```python
from build123d import *

# Parameters (mm, degrees)
BOSS_EXTRUDE1_DEPTH  = 19.9517
M3_CLEARANCE_HOLE1_D = 3.4


with BuildPart() as part:
    # Sketch1 → Boss-Extrude1 (new body)
    with BuildSketch(Plane(origin=(0, 0, 0), x_dir=(1, 0, 0), z_dir=(0, 1, 0))):
        Polygon((16.637, 24.92375), (26.67, 24.92375), (26.67, -24.92375), (16.637, -24.92375), (16.637, -32.03575), (-1.143, -32.03575), (-1.143, -24.92375), (-26.67, -24.92375), (-26.67, 24.92375), (-1.143, 24.92375), (-1.143, 32.03575), (16.637, 32.03575), align=None)
    extrude(amount=BOSS_EXTRUDE1_DEPTH)

    # M3 Clearance Hole1 (through all)
    with Locations(Plane(origin=(0, 19.9517, 0), x_dir=(1, 0, 0), z_dir=(0, 1, 0))):
        with Locations((7.747, 28.86075), (7.747, -28.86075)):
            Hole(M3_CLEARANCE_HOLE1_D / 2)


solid = part.part
```
Could you check a few things on this model? Use its own coordinates, in mm. A direction names the side the tool comes from. Round coordinates to 2 decimals unless told otherwise and drop trailing zeros. Write each loop counter-clockwise with the first axis right and the second up, starting at its lowest first coordinate (ties: lowest second). Pieces come first, ordered by that corner, then holes. Notation, with made-up numbers: M 46.25,37.25 L 81.25,37.25 A23 ccw 81.25,53.25 Z; hole C 24.25,60 d10. An arc over 180 degrees is marked long. Write each question's results on one line, items separated by ' | '. Start each with the question number.
1. Imagine slicing it at D-D on z = -26. List the corners of the cut face in (x, y) for me.
2. Imagine slicing it at C-C on x = -9. List the corners of the cut face in (y, z) for me, and give its area (3 significant figures).
3. I'm going to push flat-ended pins straight in: pin 1 Ø10 at (x, y) = (-19, 9.5) entering from -Z; pin 2 Ø10 at (x, y) = (-11, 14.5) entering from +Z; pin 3 Ø8 at (y, z) = (8.5, -29.5) entering from -X. Where does each tip first touch, or does it pass through?
4. I need wall thicknesses on L1, parallel to Z at x = 8, y = 16; L2, parallel to X at y = 1.5, z = 26.5; L3, parallel to Z at x = -23.5, y = 5.75. Which ranges of each line are inside material? Lowest first, please. Write a range as from..to.
5. Thinking about a two-plate mould opening in X: for faces 6 (the face through (6.83, 9.84, 27.43)), 7 (the face through (-1.143, 10, -28)), 8 (the face through (-14, 10, -24.924)), 9 (the face through (16.637, 10, 28)), which applies, +X half, -X half, draft (parallel to the pull), parting line (faces both ways), or undercut?
6. On a 3-axis mill with a long thin cutter (end or side, diameter ignored), from which of +Z, -Z, +X, -X, +Y, -Y can I reach the whole of each face in a straight line? I mean faces 1 (the face through (-1.143, 10, 29)), 2 (the face through (16.637, 10, -29)), 3 (the face through (-26.67, 10, 0)), 4 (the face through (22, 10, 24.924)), 5 (the face through (8, 10, -32.036)). Say none if no direction works.
7. Imagine slicing it at B-B on x = 7.5. List the corners of the cut face in (y, z) for me, and give its area (3 significant figures).
8. Imagine slicing it at A-A on y = 3.5. List the corners of the cut face in (x, z) for me, and give its area (3 significant figures).
Result sheet:
1) outline: M -1.14,0 L 16.64,0 L 16.64,19.95 L -1.14,19.95 Z
2) outline: M 0,-24.92 L 19.95,-24.92 L 19.95,24.92 L 0,24.92 Z | area: 995 mm^2
3) pin 1: stops at z = -24.92 | pin 2: stops at z = 24.92 | pin 3: stops at x = -1.14
4) L1: z = -32.04..-30.54, -27.18..27.18, 30.54..32.04 | L2: x = -1.14..16.64 | L3: z = -24.92..24.92
5) face 6: undercut | face 7: -X half | face 8: draft | face 9: +X half
6) face 1: +Z, -X, +Y, -Y | face 2: -Z, +X, +Y, -Y | face 3: +Z, -Z, -X, +Y, -Y | face 4: +Z, +X, +Y, -Y | face 5: -Z, +X, -X, +Y, -Y
7) outline: M 0,-32.04 L 19.95,-32.04 L 19.95,-30.54 L 0,-30.54 Z; M 0,-27.18 L 19.95,-27.18 L 19.95,27.18 L 0,27.18 Z; M 0,30.54 L 19.95,30.54 L 19.95,32.04 L 0,32.04 Z | area: 1,140 mm^2
8) outline: M -26.67,-24.92 L -1.14,-24.92 L -1.14,-32.04 L 16.64,-32.04 L 16.64,-24.92 L 26.67,-24.92 L 26.67,24.92 L 16.64,24.92 L 16.64,32.04 L -1.14,32.04 L -1.14,24.92 L -26.67,24.92 Z; hole C 7.75,-28.86 d3.4; hole C 7.75,28.86 d3.4 | area: 2,890 mm^2
